Work out the finished part from the listing and answer in its coordinate system (mm). Face numbers are marked on the shaded views. A direction names the side the tool comes from. Give positions to 0.01 mm unless a question says otherwise; leave off trailing zeros. Write each loop counter-clockwise with the first axis right and the second up, starting at its lowest first coordinate (ties: lowest second). Pieces come first, ordered by that corner, then holes. Notation, with made-up numbers: (10.5, -17.5) - (46.5, -17.5) arc R21 cw to (46.5, -8.5) - close; hole circle Ø2 at (-4.5, 6.5). An arc over 180 degrees is marked (long way). Write item = value, one per line.
from build123d import *

# Parameters (mm, degrees)
F1_DEPTH = 25


with BuildPart() as f1:
    # F0 (on Front) → F1 (new body)
    with BuildSketch(Plane.XZ):
        with BuildLine():
            ThreePointArc((72, 9.8), (68.280256, 18.780256), (59.3, 22.5))
            Line((59.3, 22.5), (-59.3, 22.5))
            ThreePointArc((-59.3, 22.5), (-68.280256, 18.780256), (-72, 9.8))
            Line((-72, 9.8), (-72, -22.5))
            Line((-72, -22.5), (-68, -22.5))
            ThreePointArc((-68, -22.5), (-65, -19.5), (-62, -22.5))
            Line((-62, -22.5), (-58, -22.5))
            Line((-58, -22.5), (-58, -7.5))
            Line((-58, -7.5), (-45, -7.5))
            Line((-45, -7.5), (-45, -22.5))
            Line((-45, -22.5), (45, -22.5))
            Line((45, -22.5), (45, -7.5))
            Line((45, -7.5), (58, -7.5))
            Line((58, -7.5), (58, -22.5))
            Line((58, -22.5), (62, -22.5))
            ThreePointArc((62, -22.5), (65, -19.5), (68, -22.5))
            Line((68, -22.5), (72, -22.5))
            Line((72, -22.5), (72, 9.8))
        make_face()
    extrude(amount=F1_DEPTH)


solid = f1.part
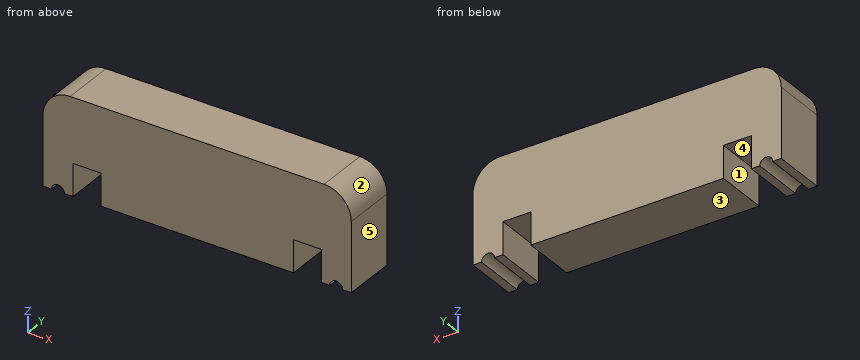
1. For a pull along X with two mould halves and no side action, classify the marked faces 3, 4 and 5 as pulls with the +X half, pulls with the -X half, needs draft (parallel to the pull), parting line crosses it, or undercut.
Solution:
face_3 = needs draft
face_4 = undercut
face_5 = pulls with the +X half
2. A tool of negligible diameter and unlimited length cuts with its end or side. For the marked faces 1 and 2, from which of +Z, -Z, +X, -X, +Y, -Y can it reach the whole face along a straight path? Write none if from no direction.
Solution:
face_1 = -Z, +Y, -Y
face_2 = +Z, +X, +Y, -Y
3. Given pin 1 (4 mm diameter, centred on x = 54, y = -14, fed in from -Z); pin 2 (10 mm diameter, centred on x = 1.5, z = -10, fed in from +Y); pin 3 (3 mm diameter, centred on y = -12, z = 17, fed in from -X); pin 4 (4 mm diameter, centred on y = -14, z = 17, fed in from +X), each flat-ended and moving along its own axis, determine where each tip first touches the part or whether it passes through.
Solution:
pin_1 = -7.5
pin_2 = 0
pin_3 = -70.65
pin_4 = 70.89
4. Find section B-B, the plane x = -50. Give the vertices of the cut face in (y, z).
Solution:
outline = (-25, -7.5) - (0, -7.5) - (0, 22.5) - (-25, 22.5) - close
5. Straight lines are drawn through the part: line 1 (X direction, y = -11, z = -17.5); line 2 (X direction, y = -4.75, z = -20); line 3 (Z direction, x = -52, y = -13.25). For each, find the intervals that lie inside material, in ascending order.
Solution:
line_1 = -72 to -58, -45 to 45, 58 to 72
line_2 = -72 to -66.66, -63.34 to -58, -45 to 45, 58 to 63.34, 66.66 to 72
line_3 = -7.5 to 22.5
6. Find section C-C, the plane x = 65. Give the vertices of the cut face in (y, z), then the cut area to 3 significant figures.
Solution:
outline = (-25, -19.5) - (0, -19.5) - (0, 21.15) - (-25, 21.15) - close
area = 1,020 mm^2
7. Find section A-A, the plane y = -20.5. Give the vertices of the cut face in (x, z).
Solution:
outline = (-72, -22.5) - (-68, -22.5) arc R3 cw to (-62, -22.5) - (-58, -22.5) - (-58, -7.5) - (-45, -7.5) - (-45, -22.5) - (45, -22.5) - (45, -7.5) - (58, -7.5) - (58, -22.5) - (62, -22.5) arc R3 cw to (68, -22.5) - (72, -22.5) - (72, 9.8) arc R12.7 ccw to (59.3, 22.5) - (-59.3, 22.5) arc R12.7 ccw to (-72, 9.8) - close
